Autodesk Inventor part; units mm, degrees
ref_plane "YZ Plane" through (0, 0, 0) normal (1, 0, 0) x (0, 1, 0)
ref_plane "XZ Plane" through (0, 0, 0) normal (0, 1, 0) x (-1, 0, 0)
ref_plane "XY Plane" through (0, 0, 0) normal (0, 0, 1) x (1, 0, 0)
sketch "Esboço1" plane through (0, 0, 0) normal (0, 1, 0) x (-1, 0, 0)
  line L0 (0, 0) -> (40, 0)
  line L1 (40, 0) -> (40, -50)
  line L2 (40, -50) -> (0, -50)
  line L3 (0, -50) -> (0, 0)
  dimension "d0" = 40
  dimension "d1" = 50
extrude "Extrusão1" add sketch "Esboço1" along normal blind 5
sketch "Esboço2" plane through (0, 5, 0) normal (0, 1, 0) x (1, 0, 0)
  line L0 (-40, 50) -> (-40, 0)
  line L1 (0, 0) -> (-40, 0)
  line L2 (-40, 0) -> (-40, 10)
  line L3 (-40, 10) -> (0, 10)
  line L4 (0, 10) -> (0, 0)
  point P0 (-40, 0)
  dimension "d4" = 10
extrude "Extrusão2" add sketch "Esboço2" along normal blind 35
sketch "Esboço3" plane through (0, 5, 0) normal (0, 1, 0) x (1, 0, 0)
  line L0 (-40, 50) -> (-40, 10)
  line L1 (0, 50) -> (-40, 50)
  point P0 (0, 0)
  point P1 (-20, 30)
  dimension "d7" = 40
  dimension "d8" = 40
  dimension "d9" = 20
  dimension "d10" = 20
hole "Furo1" at (-20, 5, -30) direction (0, -1, 0) diameter 26 end through all
sketch "Sketch4" plane through (-40, 0, 0) normal (0, 0, 1) x (1, 0, 0)
  line L0 (0, 0) -> (0, 40)
  line L1 (0, 40) -> (40, 40)
  point P0 (40, 0)
  point P1 (7.475, 12.15)
  point P2 (7.475, 32.25)
  point P3 (32.525, 12.15)
  point P4 (32.525, 32.25)
  dimension "d20" = 20.1
  dimension "d23" = 25.05
  dimension "d26" = 7.75
  dimension "d27" = 40
  dimension "d28" = 7.475
hole "Hole2" at (-32.525, 12.15, 0) at (-32.525, 32.25, 0) at (-7.475, 12.15, 0) at (-7.475, 32.25, 0) direction (0, 0, -1) diameter 5.5 end through all
equation "\"d16\" = Espessura"
equation "\"d34\" = Espessura"
equation "\"Raio_vergadura\" = Espessura"
equation "\"Largura_alívio_de_vergadura\" = Espessura"
equation "\"Profundidade_alívio_de_vergadura\" = 0.5 * Espessura"
equation "\"Tamanho_alívio_de_dobra\" = 4 * Espessura"
equation "\"Remanescente_mínimo\" = 2 * Espessura"
equation "\"Raiodetransição\" = Raio_vergadura"
equation "\"Tamanho_de_raio_de_Jacobi\" = Raio_vergadura"
equation "\"TamanhoFolga\" = Espessura"
properties part number "Suporte da guia do eixo" material "Alumínio 6061"
Here's how the part is built. I have some questions about the finished solid (model axes, mm). A direction names the side the tool comes from. Round coordinates to 2 decimals unless told otherwise and drop trailing zeros. Loops run counter-clockwise (first coordinate to the right, second up) from the corner with the lowest first, then second, coordinate; pieces in that order, holes last.
1. Which directions (+Z, -Z, +X, -X, +Y, -Y) give clear straight access to the entire face, cutting with the end or side of a thin tool? Please do faces 5 (the face through (-20, 20, 0)), 6 (the face through (-20, 5, -16)).
Answer list:
face 5: +Z, +X, -X, +Y, -Y
face 6: -Z, +X, -X, +Y
2. For P1, Ø7, axis at x = -7.475, y = 32.25, coming from the +Z side; P2, Ø1, axis at x = -27, y = 30, coming from the -Z side; P3, Ø3, axis at x = -20.5, z = -44, coming from the +Y side, each with a flat end and sliding along its axis, tell me the tip position at first contact or that it passes through.
Answer list:
P1: stops at z = 0
P2: stops at z = -10
P3: stops at y = 5
3. If we section it at C-C on y = 32.25: Write out the boundary of the cut face in (x, z) (3 decimals).
Answer list:
outline: (-40, -10) - (-35.275, -10) - (-35.275, 0) - (-40, 0) - close; (-29.775, -10) - (-10.225, -10) - (-10.225, 0) - (-29.775, 0) - close; (-4.725, -10) - (0, -10) - (0, 0) - (-4.725, 0) - close
4. If we section it at D-D on x = -25: Write out the boundary of the cut face in (y, z), plus the area to 3 significant figures.
Answer list:
outline: (0, -50) - (5, -50) - (5, -42) - (0, -42) - close; (0, -18) - (5, -18) - (5, -10) - (40, -10) - (40, 0) - (0, 0) - close
area: 480 mm2
5. If we section it at B-B on z = -25: Write out the boundary of the cut face in (x, y).
Answer list:
outline: (-40, 0) - (-32, 0) - (-32, 5) - (-40, 5) - close; (-8, 0) - (0, 0) - (0, 5) - (-8, 5) - close
6. We'd pull the mould along X, two halves only. Please class faces 1 (the face through (-20, 0, -14)), 2 (the face through (-9.794, 10.672, -5.07)), 3 (the face through (-30.85, 34.43, -5.07)), 4 (the face through (-40, 14, -8)): +X half, -X half, draft (parallel to the pull), parting line (faces both ways), or undercut.
Answer list:
face 1: draft
face 2: undercut
face 3: undercut
face 4: -X half
7. If I drill on line 1 along X through (y, z) = (32, -5); line 2 along X through (y, z) = (1.15, -30); line 3 along Y through (x, z) = (-9, -7.5), over which ranges is the centre line in solid material (lowest first)?
Answer list:
line 1: x = -40 to -35.26, -29.79 to -10.21, -4.74 to 0
line 2: x = -40 to -33, -7 to 0
line 3: y = 0 to 9.86, 14.44 to 29.96, 34.54 to 40
8. If we section it at A-A on x = -20: Write out the boundary of the cut face in (y, z).
Answer list:
outline: (0, -50) - (5, -50) - (5, -43) - (0, -43) - close; (0, -17) - (5, -17) - (5, -10) - (40, -10) - (40, 0) - (0, 0) - close
